```python
from build123d import *

# Parameters (mm, degrees)
SKETCH1_R           = 4
BOSS_EXTRUDE1_DEPTH = 52.14
SKETCH2_R           = 6
BOSS_EXTRUDE2_DEPTH = 3
CUT_EXTRUDE1_REACH  = 57.789
SKETCH3_R           = 0.2
CIRPATTERN1_COUNT   = 25


with BuildPart() as part:
    # Sketch1 → Boss-Extrude1 (new body)
    with BuildSketch(Plane(origin=(0, 0, 0), x_dir=(0, 0, -1), z_dir=(1, 0, 0))):
        Circle(SKETCH1_R)
    extrude(amount=BOSS_EXTRUDE1_DEPTH)

    # Sketch2 → Boss-Extrude2 (add)
    with BuildSketch(Plane(origin=(52.14, 0, 0), x_dir=(0, 0, -1), z_dir=(1, 0, 0))):
        Circle(SKETCH2_R)
    extrude(amount=BOSS_EXTRUDE2_DEPTH)

    # Sketch3 → Cut-Extrude1 (cut, up to next)
    with BuildSketch(Plane(origin=(55.14, 0, 0), x_dir=(0, 0, -1), z_dir=(1, 0, 0)), mode=Mode.PRIVATE) as cut_extrude1_sk1:
        with Locations((-6, 0)):
            Circle(SKETCH3_R)
    cut_extrude1_tool1 = extrude(cut_extrude1_sk1.sketch, amount=-CUT_EXTRUDE1_REACH, mode=Mode.PRIVATE) & part.part
    cut_extrude1 = cut_extrude1_tool1.solids().sort_by_distance((55.14, 0, 6))[0]
    add(cut_extrude1, mode=Mode.SUBTRACT)

    # CirPattern1: Cut-Extrude1 ×25 about axis
    cirpattern1_axis = Axis((0, 0, 0), (1, 0, 0))
    for i in range(1, CIRPATTERN1_COUNT):
        add(cut_extrude1.rotate(cirpattern1_axis, i * 360 / CIRPATTERN1_COUNT), mode=Mode.SUBTRACT)


solid = part.part
```
Verification items for the finished model (mm, model axes). A direction names the side the tool comes from. Give positions to 0.01 mm unless a question says otherwise; leave off trailing zeros. Order: outer loops, then holes, each group sorted by start corner. A loop starts at its lowest first (then second) coordinate and runs counter-clockwise, first axis right, second up. Notation, with made-up numbers: M 87,-8 L 111,-8 A23 cw 111,11 Z; hole C 25,63.25 d10. An arc over 180 degrees is marked long. Answer in a Markdown table with one row per item. Add a question column.
Item 1: Gauge pin test, flat ends, axial feed: pin 1 (2 mm diameter, centred on x = 41.5, y = -1.5, fed in from -Z); pin 2 (5 mm diameter, centred on x = 26, z = 2.5, fed in from -Y). Record the tip position at first contact, or that the pin passes through.
Item 2: Section check A-A, the plane x = 38.5. Enter the section's corners in (y, z).
Item 3: Scan lines: probe 1 along Z at (x, y) = (3, 0.5); probe 2 along X at (y, z) = (5, 1); probe 3 along Y at (x, z) = (18.5, 0). Record each from-to range of solid material in increasing order. Write a range as from..to.
Item 4: Tool access check on faces 1 (the flat face through (52.14, -3.92, 1.42)), 2 (the flat face through (55.14, 0, 0)). Record the directions out of +Z, -Z, +X, -X, +Y, -Y that give a thin tool (end or side, any length) a straight path to the whole face; none if there is none.
Filled sheet:
| question | item | result |
|---|---|---|
| 1 | pin 1 | stops at z = -3.97 |
| 1 | pin 2 | stops at y = -4 |
| 2 | outline | C 0,0 d8 |
| 3 | probe 1 | z = -3.97..3.97 |
| 3 | probe 2 | x = 52.14..55.14 |
| 3 | probe 3 | y = -4..4 |
| 4 | face 1 | -X |
| 4 | face 2 | +Z, -Z, +X, +Y, -Y |
